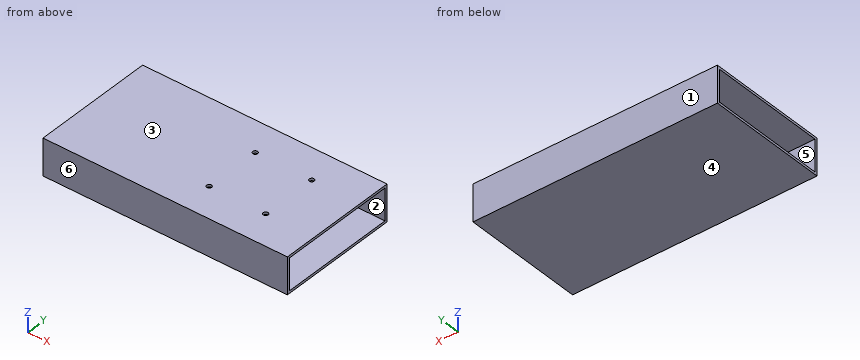
```python
from build123d import *

# Parameters (mm, degrees)
IZIM1_W                     = 400
IZIM1_H                     = 200
Y_KSEKLIK_EKSTR_ZYON2_DEPTH = 60
BO_ALTMA2_T                 = -4
KES_EKSTR_ZYON2_REACH       = 453.221
IZIM3_R                     = 4


with BuildPart() as part:
    # Çizim1 → Yükseklik-Ekstrüzyon2 (new body)
    with BuildSketch(Plane.XY):
        with Locations((-200, 100)):
            Rectangle(IZIM1_W, IZIM1_H)
    extrude(amount=Y_KSEKLIK_EKSTR_ZYON2_DEPTH)

    # İç Boşaltma2
    bo_altma2_openings = [part.faces().sort_by_distance(p)[0] for p in [
        (-400, 100, 30),
        (0, 100, 30),
    ]]
    offset(amount=BO_ALTMA2_T, openings=bo_altma2_openings, kind=Kind.INTERSECTION)

    # Çizim3 → Kes-Ekstrüzyon2 (cut, up to next)
    with BuildSketch(Plane.XY.offset(60), mode=Mode.PRIVATE) as kes_ekstr_zyon2_sk1:
        with Locations((-79.297757223, 146.25)):
            Circle(IZIM3_R)
    kes_ekstr_zyon2_tool1 = extrude(kes_ekstr_zyon2_sk1.sketch, amount=-KES_EKSTR_ZYON2_REACH, mode=Mode.PRIVATE) & part.part
    # Çizim3 → Kes-Ekstrüzyon2 (cut, up to next)
    with BuildSketch(Plane.XY.offset(60), mode=Mode.PRIVATE) as kes_ekstr_zyon2_sk2:
        with Locations((-171.797757223, 146.25)):
            Circle(IZIM3_R)
    kes_ekstr_zyon2_tool2 = extrude(kes_ekstr_zyon2_sk2.sketch, amount=-KES_EKSTR_ZYON2_REACH, mode=Mode.PRIVATE) & part.part
    # Çizim3 → Kes-Ekstrüzyon2 (cut, up to next)
    with BuildSketch(Plane.XY.offset(60), mode=Mode.PRIVATE) as kes_ekstr_zyon2_sk3:
        with Locations((-79.297757223, 53.75)):
            Circle(IZIM3_R)
    kes_ekstr_zyon2_tool3 = extrude(kes_ekstr_zyon2_sk3.sketch, amount=-KES_EKSTR_ZYON2_REACH, mode=Mode.PRIVATE) & part.part
    # Çizim3 → Kes-Ekstrüzyon2 (cut, up to next)
    with BuildSketch(Plane.XY.offset(60), mode=Mode.PRIVATE) as kes_ekstr_zyon2_sk4:
        with Locations((-171.797757223, 53.75)):
            Circle(IZIM3_R)
    kes_ekstr_zyon2_tool4 = extrude(kes_ekstr_zyon2_sk4.sketch, amount=-KES_EKSTR_ZYON2_REACH, mode=Mode.PRIVATE) & part.part
    add(kes_ekstr_zyon2_tool1.solids().sort_by_distance((-79.297757, 146.25, 60))[0], mode=Mode.SUBTRACT)
    add(kes_ekstr_zyon2_tool2.solids().sort_by_distance((-171.797757, 146.25, 60))[0], mode=Mode.SUBTRACT)
    add(kes_ekstr_zyon2_tool3.solids().sort_by_distance((-79.297757, 53.75, 60))[0], mode=Mode.SUBTRACT)
    add(kes_ekstr_zyon2_tool4.solids().sort_by_distance((-171.797757, 53.75, 60))[0], mode=Mode.SUBTRACT)


solid = part.part
```
Build history of the part. All positions in model axes, mm. Face numbers are marked on the shaded views. A direction names the side the tool comes from. Round coordinates to 2 decimals unless told otherwise and drop trailing zeros. Loops run counter-clockwise (first coordinate to the right, second up) from the corner with the lowest first, then second, coordinate; pieces in that order, holes last. Notation, with made-up numbers: M 7.5,44 L 27.5,44 A26 cw 27.5,79 Z; hole C 88,39.5 d2. An arc over 180 degrees is marked long. Answer as CSV lines item,"result".
1. Two-plate mould, pull along Z, no slides. Class the marked faces 1, 2, 3 and 4: released by +Z, released by -Z, zero draft, split by the parting line, or undercut.
Resolved:
face 1,"zero draft"
face 2,"undercut"
face 3,"released by +Z"
face 4,"released by -Z"
2. 3-axis set-ups, long thin cutter, end or side, ignore diameter. For the marked faces 5 and 6: which of +Z, -Z, +X, -X, +Y, -Y reach the whole face in a straight line?
Resolved:
face 5,"+X, -X"
face 6,"+Z, -Z, +X, -X, -Y"
3. Cut at A-A on z = 26. Write the cut outline in (x, y).
Resolved:
outline,"M -400,0 L 0,0 L 0,4 L -400,4 Z; M -400,196 L 0,196 L 0,200 L -400,200 Z"
4. Cut at C-C on x = -103. Write the cut outline in (y, z).
Resolved:
outline,"M 0,0 L 200,0 L 200,60 L 0,60 Z; hole M 4,4 L 196,4 L 196,56 L 4,56 Z"
5. Wall check: probe 1 along Z at (x, y) = (-206.5, 126); probe 2 along Y at (x, z) = (-370, 35). Give the ranges that are in metal, low to high. Write a range as [from, to].
Resolved:
probe 1,"z = [0, 4], [56, 60]"
probe 2,"y = [0, 4], [196, 200]"
6. Flat gauge pin, fed straight in: P1, Ø6, axis at x = -142.5, z = 26.5, coming from the -Y side. Where does the tip first touch, or does it go through?
Resolved:
P1,"stops at y = 0"
7. Cut at D-D on y = 90. Write the cut outline in (x, z), then the cut area to 3 significant figures.
Resolved:
outline,"M -400,0 L 0,0 L 0,4 L -400,4 Z; M -400,56 L 0,56 L 0,60 L -400,60 Z"
area,"3,200 mm²"
8. Cut at B-B on y = 146.25. Write the cut outline in (x, z), then the cut area to 3 significant figures.
Resolved:
outline,"M -400,0 L 0,0 L 0,4 L -400,4 Z; M -400,56 L -175.8,56 L -175.8,60 L -400,60 Z; M -167.8,56 L -83.3,56 L -83.3,60 L -167.8,60 Z; M -75.3,56 L 0,56 L 0,60 L -75.3,60 Z"
area,"3,140 mm²"
